Drawing for the job (mm, zero at the part's lowest x, y, z). A direction names the side the tool comes from. Round coordinates to 2 decimals unless told otherwise and drop trailing zeros. Write each loop counter-clockwise with the first axis right and the second up, starting at its lowest first coordinate (ties: lowest second). Pieces come first, ordered by that corner, then holes.
Item 1: Band-saw the part on B-B, the plane x = 20. Write the cut outline in (y, z), then the cut area to 3 significant figures.
Item 2: Wall check: probe 1 along Y at (x, z) = (10.55, 20); probe 2 along Y at (x, z) = (4.5, 32); probe 3 along Z at (x, y) = (19.5, 100). Give the ranges that are in metal, low to high.
Item 3: Drop flat-ended pins along their axis: pin 1 Ø5 at (x, z) = (17, 23.5) entering from -Y; pin 2 Ø19.5 at (y, z) = (18, 24) entering from -X; pin 3 Ø10 at (x, y) = (22, 56) entering from +Z. Give the stop position or say it passes through.
Item 4: Band-saw the part on D-D, the plane z = 27.5. Write the cut outline in (x, y).
Item 5: Band-saw the part on A-A, the plane z = 20. Write the cut outline in (x, y).
Item 6: Mould opens along X. For the marked faces 1, 2 and 3 say: +X half, -X half, draft (parallel to the pull), parting line (faces both ways), or undercut.
Item 7: 3-axis set-ups, long thin cutter, end or side, ignore diameter. For the marked faces 4 and 5: which of +Z, -Z, +X, -X, +Y, -Y reach the whole face in a straight line?
Item 8: Band-saw the part on C-C, the plane y = 22. Write the cut outline in (x, z) (1 decimal).
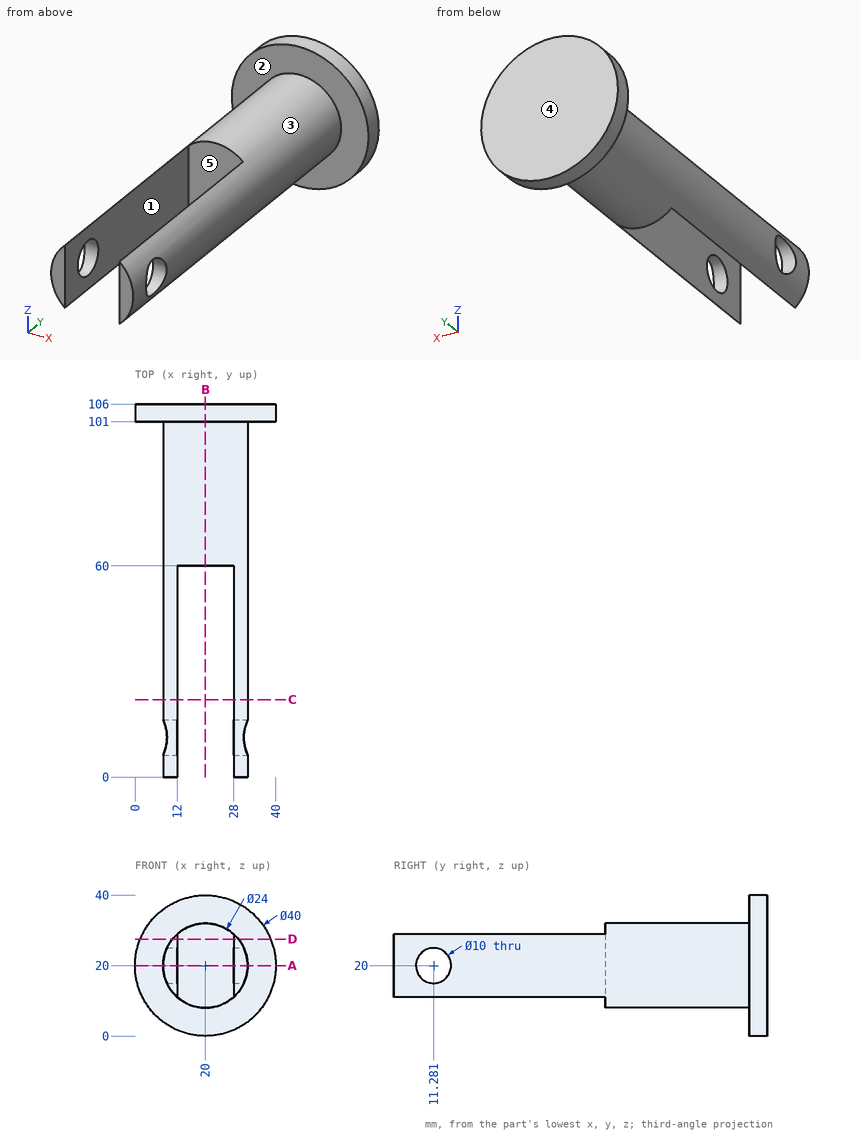
Results:
1. outline: (60, 8) - (101, 8) - (101, 0) - (106, 0) - (106, 40) - (101, 40) - (101, 32) - (60, 32) - close
1. area: 1,180 mm2
2. probe 1: y = 0 to 6.28, 16.28 to 106
2. probe 2: y = 101 to 106
2. probe 3: z = 8.01 to 31.99
3. pin 1: stops at y = 60
3. pin 2: stops at x = 8
3. pin 3: stops at z = 32
4. outline: (1.46, 101) - (10.63, 101) - (10.63, 0) - (12, 0) - (12, 60) - (28, 60) - (28, 0) - (29.37, 0) - (29.37, 101) - (38.54, 101) - (38.54, 106) - (1.46, 106) - close
5. outline: (0, 101) - (8, 101) - (8, 16.28) - (12, 16.28) - (12, 60) - (28, 60) - (28, 16.28) - (32, 16.28) - (32, 101) - (40, 101) - (40, 106) - (0, 106) - close; (8, 0) - (12, 0) - (12, 6.28) - (8, 6.28) - close; (28, 0) - (32, 0) - (32, 6.28) - (28, 6.28) - close
6. face 1: undercut
6. face 2: draft
6. face 3: parting line
7. face 4: +Z, -Z, +X, -X, +Y
7. face 5: +Z, -Z, -Y
8. outline: (12, 11.1) - (12, 28.9) arc R12 ccw to start; (28, 11.1) arc R12 ccw to (28, 28.9) - close
